from build123d import *

# Parameters (mm, degrees)
SKETCH1_R           = 2.921
BOSS_EXTRUDE1_DEPTH = 4.000000128
SKETCH2_R           = 4.2333418
BOSS_EXTRUDE2_DEPTH = 0.7499985
SKETCH3_R           = 1.05
CUT_EXTRUDE1_DEPTH  = 8.642306756
SKETCH4_R           = 2.921
CUT_EXTRUDE2_DEPTH  = 4.000000128


with BuildPart() as part:
    # Sketch1 → Boss-Extrude1 (new body)
    with BuildSketch(Plane(origin=(0, 0, 0), x_dir=(1, 0, 0), z_dir=(0, 1, 0))):
        with Locations(Location((0, 0, 0), (0, 0, 270))):
            Circle(SKETCH1_R)
    extrude(amount=BOSS_EXTRUDE1_DEPTH)

    # Sketch2 → Boss-Extrude2 (add)
    with BuildSketch(Plane(origin=(0, 4.000000128, 0), x_dir=(1, 0, 0), z_dir=(0, 1, 0))):
        with Locations(Location((0, 0, 0), (0, 0, 270))):
            Circle(SKETCH2_R)
    extrude(amount=BOSS_EXTRUDE2_DEPTH)

    # Sketch3 → Cut-Extrude1 (cut, through all)
    with BuildSketch(Plane(origin=(0, 4.749998628, 0), x_dir=(1, 0, 0), z_dir=(0, 1, 0))):
        with Locations(Location((0, 0, 0), (0, 0, 270))):
            Circle(SKETCH3_R)
    extrude(amount=-CUT_EXTRUDE1_DEPTH, mode=Mode.SUBTRACT)

    # Sketch4 → Cut-Extrude2 (cut)
    with BuildSketch(Plane.XZ):
        Circle(SKETCH4_R)
    extrude(amount=-CUT_EXTRUDE2_DEPTH, mode=Mode.SUBTRACT)


solid = part.part
Work out the finished part from the listing and answer in its coordinate system (mm). Give positions to 0.01 mm unless a question says otherwise; leave off trailing zeros. Write each loop counter-clockwise with the first axis right and the second up, starting at its lowest first coordinate (ties: lowest second). Pieces come first, ordered by that corner, then holes.
Q1. The part is cut by section A-A on x = 0. Give the vertices of the cut face in (y, z).
Answer:
outline: (4, -4.23) - (4.75, -4.23) - (4.75, -1.05) - (4, -1.05) - close; (4, 1.05) - (4.75, 1.05) - (4.75, 4.23) - (4, 4.23) - close
Q2. Straight lines are drawn through the part: L1, parallel to X at y = 4.4, z = 0; L2, parallel to X at y = 4.65, z = 0.5; L3, parallel to Z at x = 0.25, y = 4.65. For each, find the intervals that lie inside material, in ascending order.
Answer:
L1: x = -4.23 to -1.05, 1.05 to 4.23
L2: x = -4.2 to -0.92, 0.92 to 4.2
L3: z = -4.23 to -1.02, 1.02 to 4.23
Q3. The part is cut by section B-B on z = 0. Give the vertices of the cut face in (x, y), and give its area (4 significant figures).
Answer:
outline: (-4.23, 4) - (-1.05, 4) - (-1.05, 4.75) - (-4.23, 4.75) - close; (1.05, 4) - (4.23, 4) - (4.23, 4.75) - (1.05, 4.75) - close
area: 4.775 mm2
Q4. The part is cut by section C-C on y = 4.15. Give the vertices of the cut face in (x, z), and give its area (3 significant figures).
Answer:
outline: circle Ø8.47 at (0, 0); hole circle Ø2.1 at (0, 0)
area: 52.8 mm2
Q5. The part is cut by section D-D on z = -2.5. Give the vertices of the cut face in (x, y).
Answer:
outline: (-3.42, 4) - (3.42, 4) - (3.42, 4.75) - (-3.42, 4.75) - close
Q6. For a pull along Z with two mould halves and no side action, classify faces 1 (the face through (-1, 4.75, 1)), 2 (the face through (0.32, 4.38, 1)), 3 (the face through (-2.576, 4.37, -3.359)) as released by +Z, released by -Z, zero draft, split by the parting line, or undercut.
Answer:
face 1: zero draft
face 2: undercut
face 3: split by the parting line
